Model file for the job. Use its own axes, mm. Coordinates: 2 decimals unless noted, no trailing zeros. Loops run counter-clockwise (first coordinate to the right, second up) from the corner with the lowest first, then second, coordinate; pieces in that order, holes last. Notation, with made-up numbers: (-8, -6.75) -> (34, -6.75) arc R12 cw to (34, -1.75) -> close; hole circle Ø1 at (-29, -12.75). An arc over 180 degrees is marked (long way). Use one line per item in the form item = value.
Autodesk Inventor part; units mm, degrees
ref_plane "YZ Plane" through (0, 0, 0) normal (1, 0, 0) x (0, 1, 0)
ref_plane "XZ Plane" through (0, 0, 0) normal (0, 1, 0) x (-1, 0, 0)
ref_plane "XY Plane" through (0, 0, 0) normal (0, 0, 1) x (1, 0, 0)
sketch "Sketch1" plane through (0, 0, 0) normal (0, 0, 1) x (1, 0, 0)
  circle A0 centre (0, 0) radius 35
  point P0 (0, 30)
  point P1 (-25.9808, 15)
  point P2 (-25.9808, -15)
  point P3 (0, -30)
  point P4 (25.9808, -15)
  point P5 (25.9808, 15)
  dimension "d0" = 30
  dimension "d1" = 70
  dimension "d13" = 360
extrude "Extrusion1" add sketch "Sketch1" along normal blind 1.66
hole "Hole1" at (0, 30, 0) at (25.9808, 15, 0) at (0, -30, 0) at (-25.9808, -15, 0) at (-25.9808, 15, 0) at (25.9808, -15, 0) direction (0, 0, 1) diameter 3.4 depth 8 tip angle 118
properties part number "capsule.electronics.board"
Q1. Wall check: line 1 along Y through (x, z) = (0, 0.85); line 2 along Y through (x, z) = (1, 0.9); line 3 along X through (y, z) = (15, 1.3). Give the ranges that are in metal, low to high.
Result:
line_1 = -35 to -31.7, -28.3 to 28.3, 31.7 to 35
line_2 = -34.99 to -31.37, -28.63 to 28.63, 31.37 to 34.99
line_3 = -31.62 to -27.68, -24.28 to 24.28, 27.68 to 31.62
Q2. Band-saw the part on A-A, the plane x = 0. Write the cut outline in (y, z).
Result:
outline = (-35, 0) -> (-31.7, 0) -> (-31.7, 1.66) -> (-35, 1.66) -> close; (-28.3, 0) -> (28.3, 0) -> (28.3, 1.66) -> (-28.3, 1.66) -> close; (31.7, 0) -> (35, 0) -> (35, 1.66) -> (31.7, 1.66) -> close
Q3. Band-saw the part on C-C, the plane z = 0.8. Write the cut outline in (x, y).
Result:
outline = circle Ø70 at (0, 0); hole circle Ø3.4 at (-25.98, -15); hole circle Ø3.4 at (-25.98, 15); hole circle Ø3.4 at (0, -30); hole circle Ø3.4 at (0, 30); hole circle Ø3.4 at (25.98, -15); hole circle Ø3.4 at (25.98, 15)
Q4. Band-saw the part on B-B, the plane y = -30. Write the cut outline in (x, z).
Result:
outline = (-18.03, 0) -> (-1.7, 0) -> (-1.7, 1.66) -> (-18.03, 1.66) -> close; (1.7, 0) -> (18.03, 0) -> (18.03, 1.66) -> (1.7, 1.66) -> close
Q5. Band-saw the part on D-D, the plane y = -14.5. Write the cut outline in (x, z).
Result:
outline = (-31.86, 0) -> (-27.61, 0) -> (-27.61, 1.66) -> (-31.86, 1.66) -> close; (-24.36, 0) -> (24.36, 0) -> (24.36, 1.66) -> (-24.36, 1.66) -> close; (27.61, 0) -> (31.86, 0) -> (31.86, 1.66) -> (27.61, 1.66) -> close
Q6. Mould opens along Y. For faces 1 (the face through (0.65, 31.57, 0.84)), 2 (the face through (-28, 21, 1)), 3 (the face through (0, 0, 0)) say: released by +Y, released by -Y, zero draft, split by the parting line, or undercut.
Result:
face_1 = undercut
face_2 = split by the parting line
face_3 = zero draft
